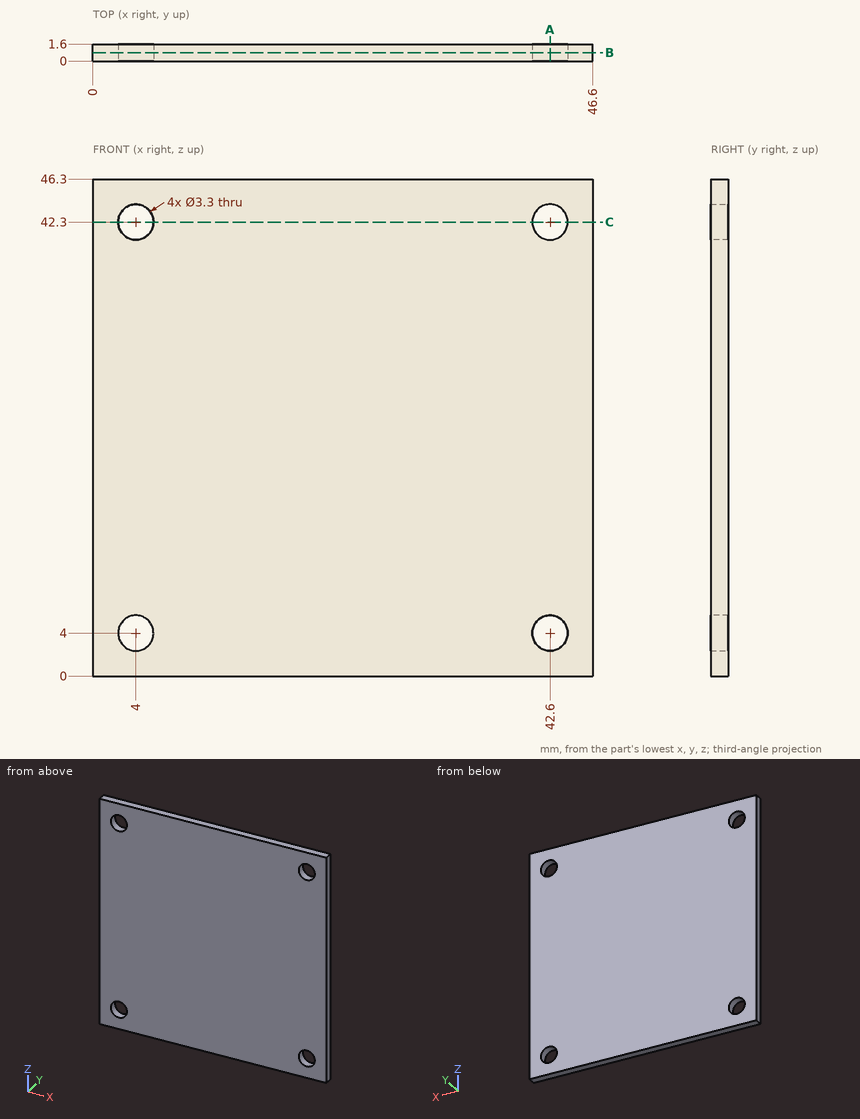
Drawing for the job (mm, zero at the part's lowest x, y, z). Give positions to 0.01 mm unless a question says otherwise; leave off trailing zeros. Order: outer loops, then holes, each group sorted by start corner. A loop starts at its lowest first (then second) coordinate and runs counter-clockwise, first axis right, second up. Notation, with made-up numbers: (42.25, 60) -> (54.25, 60) arc R14 ccw to (54.25, 74) -> close; hole circle Ø11 at (-0.5, -27). An arc over 180 degrees is marked (long way). Use one line per item in the form item = value.
(1) Saw through at B-B (y = 0.8). Write the cut outline in (x, z), then the cut area to 3 significant figures.
Solution:
outline = (0, 0) -> (46.6, 0) -> (46.6, 46.3) -> (0, 46.3) -> close; hole circle Ø3.3 at (4, 4); hole circle Ø3.3 at (4, 42.3); hole circle Ø3.3 at (42.6, 4); hole circle Ø3.3 at (42.6, 42.3)
area = 2,120 mm²
(2) Drill centre lines: line 1 (X direction, y = 1.2, z = 4); line 2 (X direction, y = 1.3, z = 41); line 3 (Z direction, x = 43.5, y = 1.05). Where is each one in solid material? Low to high. Write a range as from..to.
Solution:
line_1 = 0..2.35, 5.65..40.95, 44.25..46.6
line_2 = 0..2.98, 5.02..41.58, 43.62..46.6
line_3 = 0..2.62, 5.38..40.92, 43.68..46.3
(3) Saw through at C-C (z = 42.3). Write the cut outline in (x, y), then the cut area to 3 significant figures.
Solution:
outline = (0, 0) -> (2.35, 0) -> (2.35, 1.6) -> (0, 1.6) -> close; (5.65, 0) -> (40.95, 0) -> (40.95, 1.6) -> (5.65, 1.6) -> close; (44.25, 0) -> (46.6, 0) -> (46.6, 1.6) -> (44.25, 1.6) -> close
area = 64.0 mm²
(4) Saw through at A-A (x = 42.6). Write the cut outline in (y, z).
Solution:
outline = (0, 0) -> (1.6, 0) -> (1.6, 2.35) -> (0, 2.35) -> close; (0, 5.65) -> (1.6, 5.65) -> (1.6, 40.65) -> (0, 40.65) -> close; (0, 43.95) -> (1.6, 43.95) -> (1.6, 46.3) -> (0, 46.3) -> close
(5) Flat gauge pin, fed straight in: P1, Ø2.5, axis at x = 42.6, z = 4, coming from the -Y side. Where does the tip first touch, or does it go through?
Solution:
P1 = through
